```python
from build123d import *

# Parameters (mm, degrees)
BOSS_EXTRUDE1_DEPTH = 30.5
SKETCH4_W           = 22
SKETCH4_H           = 15
CUT_EXTRUDE2_DEPTH  = 25
CUT_EXTRUDE4_DEPTH  = 11.5
SKETCH7_W           = 31
SKETCH7_H           = 3.5
BOSS_EXTRUDE3_DEPTH = 8
BOSS_EXTRUDE4_START = -8
BOSS_EXTRUDE4_DEPTH = 8
LPATTERN1_COUNT     = 12
LPATTERN1_PITCH     = 2.5
SKETCH11_W          = 12
SKETCH11_H          = 4.5
BOSS_EXTRUDE5_DEPTH = 2
FILLET1_R           = 2
FILLET2_R           = 2
CUT_EXTRUDE5_DEPTH  = 49.427812959


with BuildPart() as part:
    # Sketch1 → Boss-Extrude1 (new body)
    with BuildSketch(Plane.XY):
        Polygon((0, 0), (0, -30), (12, -30), (12, -20), (5, 0), align=None)
    extrude(amount=-BOSS_EXTRUDE1_DEPTH)

    # Sketch4 → Cut-Extrude2 (cut)
    with BuildSketch(Plane.ZY):
        with Locations((-15.5, -22.788025353)):
            Rectangle(SKETCH4_W, SKETCH4_H)
    extrude(amount=-CUT_EXTRUDE2_DEPTH, mode=Mode.SUBTRACT)

    # Sketch6 → Cut-Extrude4 (cut, symmetric)
    with BuildSketch(Plane.XY.offset(-15.25)):
        Polygon((5, 0), (5, -14), (9.9, -14), align=None)
    extrude(amount=CUT_EXTRUDE4_DEPTH, both=True, mode=Mode.SUBTRACT)

    # Sketch7 → Boss-Extrude3 (add)
    with BuildSketch(Plane(origin=(0, -26.4, 0), x_dir=(1, 0, 0), z_dir=(0, 1, 0))):
        with Locations((-4.2231607, 27.5)):
            Rectangle(SKETCH7_W, SKETCH7_H)
    extrude(amount=BOSS_EXTRUDE3_DEPTH)

    # Sketch10 → Boss-Extrude4 (add)
    with BuildSketch(Plane(origin=(0, -18.4, 0), x_dir=(1, 0, 0), z_dir=(0, 1, 0)).offset(BOSS_EXTRUDE4_START)):
        Polygon((11.2768393, 25.75), (10.134695379, 23.01044295), (9.791251241, 23.01044295), (8.630940097, 25.75), align=None)
    boss_extrude4 = extrude(amount=BOSS_EXTRUDE4_DEPTH)

    # LPattern1: Boss-Extrude4 ×12
    with Locations(*[(-i * LPATTERN1_PITCH, 0, 0) for i in range(1, LPATTERN1_COUNT)]):
        add(boss_extrude4)

    # Sketch11 → Boss-Extrude5 (add)
    with BuildSketch(Plane(origin=(0, 0, -30.5), x_dir=(-1, 0, 0), z_dir=(0, 0, -1))):
        with Locations((-6, -27.75)):
            Rectangle(SKETCH11_W, SKETCH11_H)
    boss_extrude5 = extrude(amount=BOSS_EXTRUDE5_DEPTH)

    # Fillet1
    fillet1_edges = [part.edges().sort_by_distance(p)[0] for p in [
        (6, -25.5, -32.5),
    ]]
    fillet(fillet1_edges, radius=FILLET1_R - 0.0001)  # a hair under: the kernel refuses the full size

    # Mirror1: Boss-Extrude5 across plane
    add(boss_extrude5.mirror(Plane.XY.offset(-15.25)))

    # Fillet2
    fillet2_edges = [part.edges().sort_by_distance(p)[0] for p in [
        (6, -25.5, 2),
    ]]
    fillet(fillet2_edges, radius=FILLET2_R - 0.0001)  # a hair under: the kernel refuses the full size

    # Sketch9 → Cut-Extrude5 (cut, through all)
    with BuildSketch(Plane.ZY):
        Polygon((-6.15967028, -26.4), (-1.15967028, -26.4), (-1.15967028, -28.6), (-2.75967028, -28.6), (-2.75967028, -30.296685761), (-6.15967028, -30.296685761), align=None)
        Polygon((-27.74032972, -30.296685761), (-24.34032972, -30.296685761), (-24.34032972, -26.4), (-29.34032972, -26.4), (-29.34032972, -28.6), (-27.74032972, -28.6), align=None)
    extrude(amount=-CUT_EXTRUDE5_DEPTH, mode=Mode.SUBTRACT)


solid = part.part
```
The listing builds one solid part. Answer for the finished solid, in the listing's coordinates (mm). A direction names the side the tool comes from. Give positions to 0.01 mm unless a question says otherwise; leave off trailing zeros. Loops run counter-clockwise (first coordinate to the right, second up) from the corner with the lowest first, then second, coordinate; pieces in that order, holes last. Notation, with made-up numbers: M 64.5,-5.5 L 85.5,-5.5 A18 cw 85.5,1.5 Z; hole C -23,1 d11. An arc over 180 degrees is marked long. One line per item, written item: value.
1. For faces 1 (the face through (6, -18, -26.5)), 2 (the face through (3, 0, -15)), 3 (the face through (6, -27, -1.16)), determine the directions among +Z, -Z, +X, -X, +Y, -Y from which every point of the face is accessible in a straight line to the end or side of a thin tool.
Found:
face 1: +X
face 2: +Z, -Z, +X, -X, +Y
face 3: +X, -X
2. For a pull along Z with two mould halves and no side action, classify faces 4 (the face through (6, -10, -26.75)), 5 (the face through (10.07, -14.49, -15.18)), 6 (the face through (5.92, -26.07, -31.9)) as pulls with the +Z half, pulls with the -Z half, needs draft (parallel to the pull), parting line crosses it, or undercut.
Found:
face 4: undercut
face 5: needs draft
face 6: pulls with the -Z half
3. Section B-B on y = -9.5 is taken. Determine the outline of the cut face in (x, z) (3 decimals).
Found:
outline: M 0,-30.5 L 8.325,-30.5 L 8.325,-26.75 L 5,-26.75 L 5,-3.75 L 8.325,-3.75 L 8.325,0 L 0,0 Z
4. Each of these flat-tipped pins is pushed along its axis until it touches: P1, Ø12, axis at x = -13.5, z = -26, coming from the +Y side; P2, Ø10, axis at y = -17.5, z = -18, coming from the -X side; P3, Ø3.5, axis at x = 3.5, y = -19, coming from the -Z side; P4, Ø8, axis at y = -14.5, z = -27.5, coming from the -X side. Where does it stop, or does it pass through?
Found:
P1: y = -18.4
P2: x = 0
P3: z = -30.5
P4: x = -19.72
5. Find the intervals of material crossed by probe 1 along Y at (x, z) = (3.5, -25.5); probe 2 along Z at (x, y) = (10, -19.5); probe 3 along Z at (x, y) = (7, -10.5), in increasing order.
Found:
probe 1: -26.4 to -18.4, -15.29 to 0
probe 2: -30.5 to -23.01, -4.5 to 0
probe 3: -30.5 to -26.75, -3.75 to 0
6. Section C-C on y = -16.25 is taken. Determine the outline of the cut face in (x, z).
Found:
outline: M 0,-30.5 L 10.69,-30.5 L 10.69,-26.5 L 0,-26.5 Z; M 0,-4.5 L 10.69,-4.5 L 10.69,0 L 0,0 Z
7. Section A-A on z = -13 is taken. Determine the outline of the cut face in (x, y).
Found:
outline: M 0,-15.29 L 10.35,-15.29 L 9.9,-14 L 5,-14 L 5,0 L 0,0 Z
